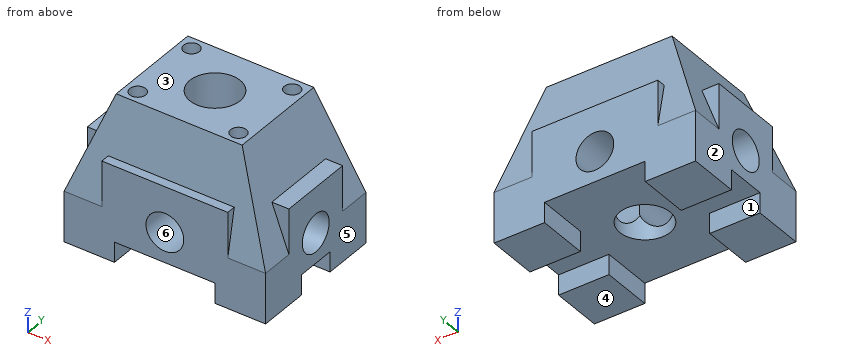
from build123d import *

# Parameters (mm, degrees)
F0_W      = 160
F0_H      = 112
F1_DEPTH  = 40
F2_W      = 80
F2_H      = 16
F3_DEPTH  = 115
F4_W      = 32
F4_H      = 16
F5_DEPTH  = 165
F6_W      = 100
F6_H      = 112
F7_DEPTH  = 36
F8_W      = 30
F8_H      = 60
F9_DEPTH  = 36
F10_W     = 30
F10_H     = 60
F11_DEPTH = 36
F14_W     = 100
F14_H     = 80
F12_W     = 160
F12_H     = 112
F16_R     = 20
F17_DEPTH = 120
F18_R     = 15
F19_DEPTH = 112
F20_R     = 15
F21_DEPTH = 160
F23_D     = 12.6
F23_DEPTH = 30
F23_TIP   = 3.7854218999


with BuildPart() as f1:
    # F0 (on Top) → F1 (new body)
    with BuildSketch(Plane.XY):
        Rectangle(F0_W, F0_H)
    extrude(amount=-F1_DEPTH)

    # F2 (on face) → F3 (cut)
    with BuildSketch(Plane.XZ.offset(56)):
        with Locations((0, -32)):
            Rectangle(F2_W, F2_H)
    extrude(amount=-F3_DEPTH, mode=Mode.SUBTRACT)

    # F4 (on face) → F5 (cut)
    with BuildSketch(Plane(origin=(-80, 0, 0), x_dir=(0, -1, 0), z_dir=(-1, 0, 0))):
        with Locations((0, -32)):
            Rectangle(F4_W, F4_H)
    extrude(amount=-F5_DEPTH, mode=Mode.SUBTRACT)

    # F6 (on face) → F7 (join)
    with BuildSketch(Plane.XY):
        Rectangle(F6_W, F6_H)
    extrude(amount=F7_DEPTH)

    # F8 (on face) → F9 (join)
    with BuildSketch(Plane.XY):
        with Locations((65, 0)):
            Rectangle(F8_W, F8_H)
    extrude(amount=F9_DEPTH)

    # F10 (on face) → F11 (join)
    with BuildSketch(Plane.XY):
        with Locations((-65, 0)):
            Rectangle(F10_W, F10_H)
    extrude(amount=F11_DEPTH)

    # F14 (on offset) → F15 section 0
    with BuildSketch(Plane.XY.offset(80)):
        Rectangle(F14_W, F14_H)
    # F12 (on Top) → F15 section 1
    with BuildSketch(Plane.XY):
        Rectangle(F12_W, F12_H)
    loft()

    # F16 (on face) → F17 (cut)
    with BuildSketch(Plane.XY.offset(80)):
        Circle(F16_R)
    extrude(amount=-F17_DEPTH, mode=Mode.SUBTRACT)

    # F18 (on face) → F19 (cut)
    with BuildSketch(Plane.XZ.offset(56)):
        Circle(F18_R)
    extrude(amount=-F19_DEPTH, mode=Mode.SUBTRACT)

    # F20 (on face) → F21 (cut)
    with BuildSketch(Plane(origin=(-80, 0, 0), x_dir=(0, -1, 0), z_dir=(-1, 0, 0))):
        Circle(F20_R)
    extrude(amount=-F21_DEPTH, mode=Mode.SUBTRACT)

    # F23
    with Locations(Plane.XY.offset(80)):
        with Locations((-40, 30), (40, 30), (40, -30), (-40, -30)):
            Hole(F23_D / 2, depth=F23_DEPTH)
            with Locations((0, 0, -(F23_DEPTH + F23_TIP / 2))):  # 118° drill point
                Cone(0, F23_D / 2, F23_TIP, mode=Mode.SUBTRACT)


solid = f1.part
Design review of the part built by this model. Coordinates are the model's own, in mm. Face numbers are marked on the shaded views. A direction names the side the tool comes from. Round coordinates to 2 decimals unless told otherwise and drop trailing zeros. Write each loop counter-clockwise with the first axis right and the second up, starting at its lowest first coordinate (ties: lowest second). Pieces come first, ordered by that corner, then holes. Notation, with made-up numbers: (44, 40.5) - (83, 40.5) arc R23 cw to (83, 57.5) - close; hole circle Ø2 at (-7, 36.25). An arc over 180 degrees is marked (long way). Use a Markdown table: item, result. Add a question column.
1. We need section B-B (y = 0). Count the separate pieces of the cut face and the enclosed holes in it, then the cut area to 3 significant figures.
2. Mouldability with a two-part tool opening along Z and no side actions: class the marked faces 3, 4, 5 and 6 as +Z half, -Z half, draft (parallel to the pull), parting line (faces both ways), or undercut.
3. Clearance check with flat-ended pins moving along their axes: pin 1 (7.5 mm diameter, centred on x = -40, y = 30, fed in from +Z); pin 2 (11.5 mm diameter, centred on x = 40, y = 30, fed in from +Z); pin 3 (4 mm diameter, centred on x = -70.5, z = 15, fed in from -Y). State where each tip first meets the part, or that it passes through.
4. For the marked faces 1 and 2, list the 3-axis set-ups (+Z, -Z, +X, -X, +Y, -Y) from which the entire face can be reached by the end or side of a thin tool; tool diameter is ignored.
5. Wall thickness on probe 1 along Y at (x, z) = (-40, 72.25); probe 2 along Z at (x, y) = (-43.5, 0); probe 3 along X at (y, z) = (44.5, 0): over which ranges is each line inside the solid? List them lowest first.
6. We need section A-A (z = -26). State the section outline as (x, y) points.
Output:
| question | item | result |
|---|---|---|
| 1 | separate pieces | 4 |
| 1 | enclosed holes | 0 |
| 1 | area | 6,970 mm2 |
| 2 | face 3 | +Z half |
| 2 | face 4 | -Z half |
| 2 | face 5 | draft |
| 2 | face 6 | undercut |
| 3 | pin 1 | stops at z = 48.47 |
| 3 | pin 2 | stops at z = 49.67 |
| 3 | pin 3 | stops at y = -53.4 |
| 4 | face 1 | -Z, +X, -X |
| 4 | face 2 | +Z, -Z, -X, +Y, -Y |
| 5 | probe 1 | y = -41.55 to -36.3, -23.7 to 23.7, 36.3 to 41.55 |
| 5 | probe 2 | z = -24 to -15, 15 to 80 |
| 5 | probe 3 | x = -80 to -15, 15 to 80 |
| 6 | outline | (-80, -56) - (-40, -56) - (-40, -16) - (-80, -16) - close; (-80, 16) - (-40, 16) - (-40, 56) - (-80, 56) - close; (40, -56) - (80, -56) - (80, -16) - (40, -16) - close; (40, 16) - (80, 16) - (80, 56) - (40, 56) - close |
